Verification items for the finished model (mm, model axes). Face numbers are marked on the shaded views. A direction names the side the tool comes from. Round coordinates to 2 decimals unless told otherwise and drop trailing zeros. Order: outer loops, then holes, each group sorted by start corner. A loop starts at its lowest first (then second) coordinate and runs counter-clockwise, first axis right, second up. Notation, with made-up numbers: (54, 75.25) -> (74, 75.25) arc R22 cw to (74, 107.25) -> close; hole circle Ø4 at (29, 27.5). An arc over 180 degrees is marked (long way). Put each result on its own line as item: value.
```python
from build123d import *

# Parameters (mm, degrees)
F0_W     = 13
F0_H     = 11
F1_DEPTH = 16
F2_W     = 11
F2_H     = 7
F3_DEPTH = 6
F4_R     = 0.5
F5_R     = 0.5
F6_DEPTH = 1
F7_DEPTH = 3
F9_DEPTH = 0.6
F10_R    = 0.3


# Not quite as in the source:
# - a feature names something its author has since deleted; it is built from what else it names


with BuildPart() as f1:
    # F0 (on Top) → F1 (new body)
    with BuildSketch(Plane.XY):
        with Locations((6.5, 5.5)):
            Rectangle(F0_W, F0_H)
    extrude(amount=F1_DEPTH)

    # F2 (on face) → F3 (cut)
    with BuildSketch(Plane.XY.offset(16)):
        with Locations((6.5, 6.5)):
            Rectangle(F2_W, F2_H)
    extrude(amount=-F3_DEPTH, mode=Mode.SUBTRACT)

    # F4
    f4_edges = [f1.edges().sort_by_distance(p)[0] for p in [
        (1, 6.5, 10),
        (6.5, 3, 10),
        (12, 6.5, 10),
        (6.5, 10, 10),
    ]]
    fillet(f4_edges, radius=F4_R)

    # F5 (on face) → F6 (join)
    with BuildSketch(Plane.XY.offset(16)):
        with Locations((5, 2)):
            Circle(F5_R)
        with Locations((8, 2)):
            Circle(F5_R)
    extrude(amount=F6_DEPTH)

    # F5 (on face) → F7 (join)
    with BuildSketch(Plane.XY.offset(16)):
        with Locations((6.5, 2)):
            Circle(F5_R)
    extrude(amount=F7_DEPTH)

    # F8 (on face) → F9 (join)
    with BuildSketch(Plane.XY.offset(19)):
        with BuildLine():
            Line((6, 5), (6, 2))
            ThreePointArc((6, 2), (6.5, 1.5), (7, 2))
            Line((7, 2), (7, 5))
            ThreePointArc((7, 5), (6.5, 5.5), (6, 5))
        make_face()
    extrude(amount=F9_DEPTH)

    # F10
    f10_edges = [f1.edges().sort_by_distance(p)[0] for p in [
        (6, 3.5, 19.6),
        (6.5, 1.5, 19.6),
        (7, 3.5, 19.6),
        (6.5, 5.5, 19.6),
    ]]
    fillet(f10_edges, radius=F10_R)


solid = f1.part
```
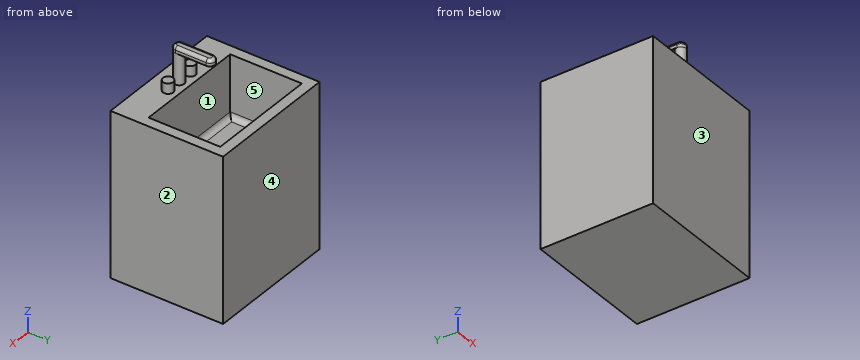
Item 1: Sectioned sample at A-A, the plane y = 3.75. Record the boundary of the cut face in (x, z).
Geometry check:
outline: (0, 0) -> (13, 0) -> (13, 16) -> (12, 16) -> (12, 10.5) arc R0.5 cw to (11.5, 10) -> (1.5, 10) arc R0.5 cw to (1, 10.5) -> (1, 16) -> (0, 16) -> close; (6, 19) -> (7, 19) -> (7, 19.3) arc R0.3 ccw to (6.7, 19.6) -> (6.3, 19.6) arc R0.3 ccw to (6, 19.3) -> close
Item 2: Tool access check on the marked faces 4 and 5. Record the directions out of +Z, -Z, +X, -X, +Y, -Y that give a thin tool (end or side, any length) a straight path to the whole face; none if there is none.
Geometry check:
face 4: +Z, -Z, +X, -X, +Y
face 5: +Z
Item 3: Material ranges on line 1 along Z through (x, y) = (2.25, 8); line 2 along X through (y, z) = (6.5, 14.25); line 3 along Z through (x, y) = (10, 2.5), recorded low to high.
Geometry check:
line 1: 0 to 10
line 2: 0 to 1, 12 to 13
line 3: 0 to 16
Item 4: Sectioned sample at B-B, the plane x = 5. Record the boundary of the cut face in (y, z), then the cut area to 3 significant figures.
Geometry check:
outline: (0, 0) -> (11, 0) -> (11, 16) -> (10, 16) -> (10, 10.5) arc R0.5 cw to (9.5, 10) -> (3.5, 10) arc R0.5 cw to (3, 10.5) -> (3, 16) -> (2.5, 16) -> (2.5, 17) -> (1.5, 17) -> (1.5, 16) -> (0, 16) -> close
area: 135 mm2
Item 5: Release check for a two-part mould opening along X. For the marked faces 1, 2 and 3 record: pulls with the +X half, pulls with the -X half, needs draft (parallel to the pull), parting line crosses it, or undercut.
Geometry check:
face 1: undercut
face 2: pulls with the +X half
face 3: needs draft
Item 6: Sectioned sample at D-D, the plane z = 18.5. Record the boundary of the cut face in (x, y).
Geometry check:
outline: circle Ø1 at (6.5, 2)
Item 7: Sectioned sample at C-C, the plane y = 8.75. Record the boundary of the cut face in (x, z).
Geometry check:
outline: (0, 0) -> (13, 0) -> (13, 16) -> (12, 16) -> (12, 10.5) arc R0.5 cw to (11.5, 10) -> (1.5, 10) arc R0.5 cw to (1, 10.5) -> (1, 16) -> (0, 16) -> close
Item 8: Depth check by flat-ended pin: pin 1 Ø1.1 at (x, y) = (8, 2) entering from +Z; pin 2 Ø5 at (x, y) = (11, 2.5) entering from +Z. Enter the tip coordinate at first touch or a pass-through.
Geometry check:
pin 1: z = 17
pin 2: z = 16
